from build123d import *

# Parameters (mm, degrees)
SKICA2_R                = 2.1
SKICA2_W                = 3
SKICA2_H                = 20
SKICA2_H_2              = 10
SKICA2_W_2              = 20
SKICA2_H_3              = 3
SKICA2_W_3              = 15
SKICA2_W_4              = 155
SKICA2_H_4              = 53
SKICA2_W_5              = 120
SKICA2_H_5              = 120
P_IDAT_VYSUNUT_M1_DEPTH = 3


with BuildPart() as part:
    # Skica2 → Přidat vysunutím1 (new body)
    with BuildSketch(Plane.XY):
        Polygon((-117.5, 80), (-77.5, 120), (77.5, 120), (117.5, 80), (117.5, -80), (77.5, -120), (-77.5, -120), (-117.5, -80), align=None)
        with Locations((14.611145618, 38.425)):
            Circle(SKICA2_R, mode=Mode.SUBTRACT)
        with Locations((14.611145618, 28.575)):
            Circle(SKICA2_R, mode=Mode.SUBTRACT)
        with Locations((-34.811145618, 28.575)):
            Circle(SKICA2_R, mode=Mode.SUBTRACT)
        with Locations((-34.811145618, 38.425)):
            Circle(SKICA2_R, mode=Mode.SUBTRACT)
        with Locations((-112.5, 70)):
            Rectangle(SKICA2_W, SKICA2_H, mode=Mode.SUBTRACT)
        with Locations((-112.5, 30)):
            Rectangle(SKICA2_W, SKICA2_H, mode=Mode.SUBTRACT)
        with Locations((-112.5, 0)):
            Rectangle(SKICA2_W, SKICA2_H_2, mode=Mode.SUBTRACT)
        with Locations((-112.5, -30)):
            Rectangle(SKICA2_W, SKICA2_H, mode=Mode.SUBTRACT)
        with Locations((-112.5, -70)):
            Rectangle(SKICA2_W, SKICA2_H, mode=Mode.SUBTRACT)
        with Locations((112.5, -70)):
            Rectangle(SKICA2_W, SKICA2_H, mode=Mode.SUBTRACT)
        with Locations((112.5, -30)):
            Rectangle(SKICA2_W, SKICA2_H, mode=Mode.SUBTRACT)
        with Locations((112.5, 0)):
            Rectangle(SKICA2_W, SKICA2_H_2, mode=Mode.SUBTRACT)
        with Locations((112.5, 30)):
            Rectangle(SKICA2_W, SKICA2_H, mode=Mode.SUBTRACT)
        with Locations((112.5, 70)):
            Rectangle(SKICA2_W, SKICA2_H, mode=Mode.SUBTRACT)
        with Locations((-67.5, 115)):
            Rectangle(SKICA2_W_2, SKICA2_H_3, mode=Mode.SUBTRACT)
        with Locations((-32.5, 115)):
            Rectangle(SKICA2_W_2, SKICA2_H_3, mode=Mode.SUBTRACT)
        with Locations((0, 115)):
            Rectangle(SKICA2_W_3, SKICA2_H_3, mode=Mode.SUBTRACT)
        with Locations((32.5, 115)):
            Rectangle(SKICA2_W_2, SKICA2_H_3, mode=Mode.SUBTRACT)
        with Locations((67.5, 115)):
            Rectangle(SKICA2_W_2, SKICA2_H_3, mode=Mode.SUBTRACT)
        with Locations((67.5, -115)):
            Rectangle(SKICA2_W_2, SKICA2_H_3, mode=Mode.SUBTRACT)
        with Locations((32.5, -115)):
            Rectangle(SKICA2_W_2, SKICA2_H_3, mode=Mode.SUBTRACT)
        with Locations((0, -115)):
            Rectangle(SKICA2_W_3, SKICA2_H_3, mode=Mode.SUBTRACT)
        with Locations((-32.5, -115)):
            Rectangle(SKICA2_W_2, SKICA2_H_3, mode=Mode.SUBTRACT)
        with Locations((-67.5, -115)):
            Rectangle(SKICA2_W_2, SKICA2_H_3, mode=Mode.SUBTRACT)
        Polygon((101.168524548, -91.381727984), (88.881727984, -103.668524548), (86.76040764, -101.547204204), (99.047204204, -89.26040764), align=None, mode=Mode.SUBTRACT)
        Polygon((-86.76040764, -101.547204204), (-99.047204204, -89.26040764), (-101.168524548, -91.381727984), (-88.881727984, -103.668524548), align=None, mode=Mode.SUBTRACT)
        Polygon((86.76040764, 101.547204204), (99.047204204, 89.26040764), (101.168524548, 91.381727984), (88.881727984, 103.668524548), align=None, mode=Mode.SUBTRACT)
        Polygon((-88.881727984, 103.668524548), (-86.76040764, 101.547204204), (-99.047204204, 89.26040764), (-101.168524548, 91.381727984), align=None, mode=Mode.SUBTRACT)
        with Locations((0, 77)):
            Rectangle(SKICA2_W_4, SKICA2_H_4, mode=Mode.SUBTRACT)
        with Locations((0, -43.5)):
            Rectangle(SKICA2_W_5, SKICA2_H_5, mode=Mode.SUBTRACT)
        Polygon((-30.05, 43.35), (-30.05, 33.975), (-36.6, 33.975), (-36.6, 33.025), (-30.05, 33.025), (-30.05, 23.65), (9.85, 23.65), (9.85, 33.025), (16.4, 33.025), (16.4, 33.975), (9.85, 33.975), (9.85, 43.35), align=None, mode=Mode.SUBTRACT)
    extrude(amount=P_IDAT_VYSUNUT_M1_DEPTH)


solid = part.part
Work out the finished part from the listing and answer in its coordinate system (mm). A direction names the side the tool comes from. Give positions to 0.01 mm unless a question says otherwise; leave off trailing zeros. Loops run counter-clockwise (first coordinate to the right, second up) from the corner with the lowest first, then second, coordinate; pieces in that order, holes last. Notation, with made-up numbers: M 3.25,35 L 49.25,35 A24 cw 49.25,65 Z; hole C 38,83 d5. An arc over 180 degrees is marked long. Use CSV: the item, a comma, the result in double quotes.
1) Find section A-A on y = -55.5. Write down the section's boundary in (x, z), plus the area to 3 significant figures.
Answer:
outline,"M -117.5,0 L -60,0 L -60,3 L -117.5,3 Z; M 60,0 L 117.5,0 L 117.5,3 L 60,3 Z"
area,"345 mm^2"
2) Determine the mould class of faces 1 (the flat face through (-92.82, -95.49, 1.48)), 2 (the flat face through (95.11, -97.44, 1.48)), 3 (the flat face through (28, 28, 3)), 4 (the flat face through (-97.2, -100.3, 1.5)) for opening direction X: released by +X, released by -X, zero draft, split by the parting line, or undercut.
Answer:
face 1,"undercut"
face 2,"undercut"
face 3,"zero draft"
face 4,"released by -X"
3) Find section C-C on x = 1.5. Write down the section's boundary in (y, z), plus the area to 3 significant figures.
Answer:
outline,"M -120,0 L -116.5,0 L -116.5,3 L -120,3 Z; M -113.5,0 L -103.5,0 L -103.5,3 L -113.5,3 Z; M 16.5,0 L 23.65,0 L 23.65,3 L 16.5,3 Z; M 43.35,0 L 50.5,0 L 50.5,3 L 43.35,3 Z; M 103.5,0 L 113.5,0 L 113.5,3 L 103.5,3 Z; M 116.5,0 L 120,0 L 120,3 L 116.5,3 Z"
area,"124 mm^2"
4) Find section B-B on y = 1. Write down the section's boundary in (x, z).
Answer:
outline,"M -117.5,0 L -114,0 L -114,3 L -117.5,3 Z; M -111,0 L -60,0 L -60,3 L -111,3 Z; M 60,0 L 111,0 L 111,3 L 60,3 Z; M 114,0 L 117.5,0 L 117.5,3 L 114,3 Z"
5) Consider L1, parallel to Y at x = -76, z = 2.5; L2, parallel to Y at x = 45, z = 2.55; L3, parallel to X at y = 66, z = 2.05. Determine where each line is inside the solid, lowest interval first.
Answer:
L1,"-120 to -116.5, -113.5 to 50.5, 103.5 to 113.5, 116.5 to 120"
L2,"-120 to -103.5, 16.5 to 50.5, 103.5 to 120"
L3,"-117.5 to -114, -111 to -77.5, 77.5 to 111, 114 to 117.5"
6) Which of the six approach directions +Z, -Z, +X, -X, +Y, -Y give full straight-line access (tool end or side, diameter ignored) to faces 5 (the flat face through (-95.11, 97.44, 1.48)), 6 (the flat face through (97.2, 100.3, 1.5))?
Answer:
face 5,"+Z, -Z"
face 6,"+Z, -Z, +X, +Y"
7) Find section D-D on y = 55. Write down the section's boundary in (x, z).
Answer:
outline,"M -117.5,0 L -77.5,0 L -77.5,3 L -117.5,3 Z; M 77.5,0 L 117.5,0 L 117.5,3 L 77.5,3 Z"
